```python
from build123d import *

# Parameters (mm, degrees)
F0_R     = 44
F1_DEPTH = 2.5
F2_R     = 10


# Not quite as in the source:
# - a feature names something its author has since deleted; it is built from what else it names


with BuildPart() as f1:
    # F0 (on Top) → F1 (new body)
    with BuildSketch(Plane.XY):
        with BuildLine():
            ThreePointArc((52.3444859472, -16.8835657052), (54.3320657029, -8.5455623836), (55, 0))
            ThreePointArc((55, 0), (54.3320657029, 8.5455623836), (52.3444859472, 16.8835657052))
            ThreePointArc((52.3444859472, 16.8835657052), (50.268991125, 22.3165528538), (47.6313971166, 27.5000001585))
            ThreePointArc((47.6313971166, 27.5000001585), (44.461197151, 32.3759470579), (40.7938397808, 36.8898717257))
            ThreePointArc((40.7938397808, 36.8898717257), (27.5, 47.6313972081), (11.5506461665, 53.7734374309))
            ThreePointArc((11.5506461665, 53.7734374309), (5.8077939557, 54.6924997542), (-3e-09, 55))
            ThreePointArc((-3e-09, 55), (-5.8077939587, 54.6924997539), (-11.5506461665, 53.7734374309))
            ThreePointArc((-11.5506461665, 53.7734374309), (-27.5, 47.6313972081), (-40.7938397808, 36.8898717257))
            ThreePointArc((-40.7938397808, 36.8898717257), (-44.4611971512, 32.3759470576), (-47.631397117, 27.5000001579))
            ThreePointArc((-47.631397117, 27.5000001579), (-50.2689911251, 22.3165528534), (-52.3444859472, 16.8835657052))
            ThreePointArc((-52.3444859472, 16.8835657052), (-55, 0), (-52.3444859472, -16.8835657052))
            ThreePointArc((-52.3444859472, -16.8835657052), (-50.2689910436, -22.3165530371), (-47.631396916, -27.500000506))
            ThreePointArc((-47.631396916, -27.500000506), (-44.4611970329, -32.3759472201), (-40.7938397808, -36.8898717257))
            ThreePointArc((-40.7938397808, -36.8898717257), (-27.5, -47.6313972081), (-11.5506461665, -53.7734374309))
            ThreePointArc((-11.5506461665, -53.7734374309), (-5.8077939898, -54.6924997506), (-6.55e-08, -55))
            ThreePointArc((-6.55e-08, -55), (5.8077939247, -54.6924997575), (11.5506461665, -53.7734374309))
            ThreePointArc((11.5506461665, -53.7734374309), (27.5, -47.6313972081), (40.7938397808, -36.8898717257))
            ThreePointArc((40.7938397808, -36.8898717257), (44.461197297, -32.3759468575), (47.6313973645, -27.4999997291))
            ThreePointArc((47.6313973645, -27.4999997291), (50.2689912256, -22.3165526272), (52.3444859472, -16.8835657052))
        make_face()
        Circle(F0_R, mode=Mode.SUBTRACT)
        with BuildLine():
            ThreePointArc((-3e-09, 55), (5.8077939557, 54.6924997542), (11.5506461665, 53.7734374309))
            Line((11.5506461665, 53.7734374309), (9.7805788286, 62.0833333333))
            ThreePointArc((9.7805788286, 62.0833333333), (0, 70), (-9.7805788286, 62.0833333333))
            Line((-9.7805788286, 62.0833333333), (-11.5506461665, 53.7734374309))
            ThreePointArc((-11.5506461665, 53.7734374309), (-5.8077939587, 54.6924997539), (-3e-09, 55))
        make_face()
        with BuildLine():
            ThreePointArc((5, 60), (3.5355339049, 56.464466093), (-3e-09, 55))
            ThreePointArc((-3e-09, 55), (-3.5355339049, 63.535533907), (5, 60))
        make_face(mode=Mode.SUBTRACT)
        with BuildLine():
            ThreePointArc((-47.631397117, 27.5000001579), (-44.4611971512, 32.3759470576), (-40.7938397808, 36.8898717257))
            Line((-40.7938397808, 36.8898717257), (-48.875454404, 39.5118963959))
            ThreePointArc((-48.875454404, 39.5118963959), (-60.6217782649, 35), (-58.6560332326, 22.5714369374))
            Line((-58.6560332326, 22.5714369374), (-52.3444859472, 16.8835657052))
            ThreePointArc((-52.3444859472, 16.8835657052), (-50.2689911251, 22.3165528534), (-47.631397117, 27.5000001579))
        make_face()
        with BuildLine():
            ThreePointArc((-46.9615242271, 30), (-47.131895072, 28.7059048625), (-47.631397117, 27.5000001579))
            ThreePointArc((-47.631397117, 27.5000001579), (-56.7911533821, 31.2940951375), (-46.9615242271, 30))
        make_face(mode=Mode.SUBTRACT)
        with BuildLine():
            Line((-48.875454404, -39.5118963959), (-40.7938397808, -36.8898717257))
            ThreePointArc((-40.7938397808, -36.8898717257), (-44.4611970329, -32.3759472201), (-47.631396916, -27.500000506))
            ThreePointArc((-47.631396916, -27.500000506), (-50.2689910436, -22.3165530371), (-52.3444859472, -16.8835657052))
            Line((-52.3444859472, -16.8835657052), (-58.6560332326, -22.5714369374))
            ThreePointArc((-58.6560332326, -22.5714369374), (-60.6217782649, -35), (-48.875454404, -39.5118963959))
        make_face()
        with BuildLine():
            ThreePointArc((-46.9615242271, -30), (-56.7911534341, -31.2940949433), (-47.631396916, -27.500000506))
            ThreePointArc((-47.631396916, -27.500000506), (-47.13189502, -28.7059050567), (-46.9615242271, -30))
        make_face(mode=Mode.SUBTRACT)
        with BuildLine():
            Line((9.7805788286, -62.0833333333), (11.5506461665, -53.7734374309))
            ThreePointArc((11.5506461665, -53.7734374309), (5.8077939247, -54.6924997575), (-6.55e-08, -55))
            ThreePointArc((-6.55e-08, -55), (-5.8077939898, -54.6924997506), (-11.5506461665, -53.7734374309))
            Line((-11.5506461665, -53.7734374309), (-9.7805788286, -62.0833333333))
            ThreePointArc((-9.7805788286, -62.0833333333), (0, -70), (9.7805788286, -62.0833333333))
        make_face()
        with BuildLine():
            ThreePointArc((5, -60), (-3.5355338828, -63.5355339291), (-6.55e-08, -55))
            ThreePointArc((-6.55e-08, -55), (3.5355338828, -56.4644660709), (5, -60))
        make_face(mode=Mode.SUBTRACT)
        with BuildLine():
            Line((58.6560332326, -22.5714369374), (52.3444859472, -16.8835657052))
            ThreePointArc((52.3444859472, -16.8835657052), (50.2689912256, -22.3165526272), (47.6313973645, -27.4999997291))
            ThreePointArc((47.6313973645, -27.4999997291), (44.461197297, -32.3759468575), (40.7938397808, -36.8898717257))
            Line((40.7938397808, -36.8898717257), (48.875454404, -39.5118963959))
            ThreePointArc((48.875454404, -39.5118963959), (60.6217782649, -35), (58.6560332326, -22.5714369374))
        make_face()
        with BuildLine():
            ThreePointArc((56.9615242271, -30), (50.6674288505, -34.829629091), (47.6313973645, -27.4999997291))
            ThreePointArc((47.6313973645, -27.4999997291), (53.2556196037, -25.170370909), (56.9615242271, -30))
        make_face(mode=Mode.SUBTRACT)
        with BuildLine():
            ThreePointArc((47.6313971166, 27.5000001585), (50.268991125, 22.3165528538), (52.3444859472, 16.8835657052))
            Line((52.3444859472, 16.8835657052), (58.6560332326, 22.5714369374))
            ThreePointArc((58.6560332326, 22.5714369374), (60.6217782649, 35), (48.875454404, 39.5118963959))
            Line((48.875454404, 39.5118963959), (40.7938397808, 36.8898717257))
            ThreePointArc((40.7938397808, 36.8898717257), (44.461197151, 32.3759470579), (47.6313971166, 27.5000001585))
        make_face()
        with BuildLine():
            ThreePointArc((56.9615242271, 30), (53.2556193642, 25.1703708449), (47.6313971166, 27.5000001585))
            ThreePointArc((47.6313971166, 27.5000001585), (50.66742909, 34.8296291551), (56.9615242271, 30))
        make_face(mode=Mode.SUBTRACT)
    extrude(amount=F1_DEPTH)

    # F2
    f2_edges = [f1.edges().sort_by_distance(p)[0] for p in [
        (52.344486, -16.883566, 1.25),
        (52.344486, 16.883566, 1.25),
        (40.79384, 36.889872, 1.25),
        (11.550646, 53.773437, 1.25),
        (-11.550646, 53.773437, 1.25),
        (-40.79384, 36.889872, 1.25),
        (-52.344486, 16.883566, 1.25),
        (-52.344486, -16.883566, 1.25),
        (-40.79384, -36.889872, 1.25),
        (-11.550646, -53.773437, 1.25),
        (11.550646, -53.773437, 1.25),
        (40.79384, -36.889872, 1.25),
    ]]
    fillet(f2_edges, radius=F2_R)


solid = f1.part
```
Here's how the part is built. I have some questions about the finished solid (model axes, mm). Coordinates: 2 decimals unless noted, no trailing zeros. Write each loop counter-clockwise with the first axis right and the second up, starting at its lowest first coordinate (ties: lowest second). Pieces come first, ordered by that corner, then holes. Notation, with made-up numbers: (62.5, -21) -> (116.5, -21) arc R24 ccw to (116.5, 2) -> close; hole circle Ø4 at (54, 72). An arc over 180 degrees is marked (long way). Use a Markdown table: item, result. Add a question column.
(1) If we section it at A-A, the plane y = 4.5: Write out the boundary of the cut face in (x, z), and give its area (3 significant figures).
(2) If we section it at D-D, the plane y = 33.5: Write out the boundary of the cut face in (x, z).
(3) If we section it at C-C, the plane z = 1.5: State how many separate pieces and enclosed holes the cut face has, and give its area (3 significant figures).
(4) Please list where these lines run through material, in increasing order: line 1 (Y direction, x = 0, z = 1.3); line 2 (Y direction, x = -50, z = 0.6); line 3 (X direction, y = -30, z = 1.35).
(5) I'm going to push flat-ended pins straight in: P1, Ø9, axis at x = -51.96, y = -30, coming from the -Z side (3 decimals); P2, Ø1.5, axis at x = 14, z = 0.5, coming from the -Y side. Where does each tip first touch, or does it pass through?
(6) If we section it at B-B, the plane x = 25: Write out the boundary of the cut face in (y, z).
(7) We'd pull the mould along Y, two halves only. Please class faces 1 (the cylindrical face through (-54.085, -16.697, 1.268)), 2 (the cylindrical face through (0, 70, 1)), 3 (the cylindrical face through (27.36, -47.71, 1.23)): +Y half, -Y half, draft (parallel to the pull), parting line (faces both ways), or undercut.
Outcome:
| question | item | result |
|---|---|---|
| 1 | outline | (-54.82, 0) -> (-43.77, 0) -> (-43.77, 2.5) -> (-54.82, 2.5) -> close; (43.77, 0) -> (54.82, 0) -> (54.82, 2.5) -> (43.77, 2.5) -> close |
| 1 | area | 55.2 mm^2 |
| 2 | outline | (-61.33, 0) -> (-55.53, 0) -> (-55.53, 2.5) -> (-61.33, 2.5) -> close; (-48.39, 0) -> (-28.53, 0) -> (-28.53, 2.5) -> (-48.39, 2.5) -> close; (28.53, 0) -> (48.39, 0) -> (48.39, 2.5) -> (28.53, 2.5) -> close; (55.53, 0) -> (61.33, 0) -> (61.33, 2.5) -> (55.53, 2.5) -> close |
| 3 | separate pieces | 1 |
| 3 | enclosed holes | 7 |
| 3 | area | 4,670 mm^2 |
| 4 | line 1 | y = -70 to -65, -55 to -44, 44 to 55, 65 to 70 |
| 4 | line 2 | y = -39.81 to -34.6, -25.4 to 25.4, 34.6 to 39.81 |
| 4 | line 3 | x = -61.96 to -56.96, -46.96 to -32.19, 32.19 to 46.96, 56.96 to 61.96 |
| 5 | P1 | passes through |
| 5 | P2 | stops at y = -54.5 |
| 6 | outline | (-48.99, 0) -> (-36.21, 0) -> (-36.21, 2.5) -> (-48.99, 2.5) -> close; (36.21, 0) -> (48.99, 0) -> (48.99, 2.5) -> (36.21, 2.5) -> close |
| 7 | face 1 | undercut |
| 7 | face 2 | +Y half |
| 7 | face 3 | -Y half |
